The listing builds one solid part. Answer for the finished solid, in the listing's coordinates (mm). A direction names the side the tool comes from. Round coordinates to 2 decimals unless told otherwise and drop trailing zeros. Write each loop counter-clockwise with the first axis right and the second up, starting at its lowest first coordinate (ties: lowest second). Pieces come first, ordered by that corner, then holes. Notation, with made-up numbers: (28.5, 30) - (38.5, 30) arc R29 cw to (38.5, 67) - close; hole circle Ø5 at (52.5, 16.5). An arc over 180 degrees is marked (long way). Return JSON: item names as keys, results as strings. Group by question number.
(1) Each of these flat-tipped pins is pushed along its axis until it touches: pin 1 (3 mm diameter, centred on x = -20.5, z = 12.5, fed in from -Y); pin 2 (6 mm diameter, centred on x = -13, z = 32.5, fed in from -Y); pin 3 (1.7 mm diameter, centred on y = -5.5, z = 8, fed in from +X); pin 4 (5 mm diameter, centred on y = -9.5, z = 17, fed in from -X). Where does it stop, or does it pass through?
(2) Section A-A, the plane x = -32 is taken. Write down the section's boundary in (y, z), then the cut area to 3 significant figures.
(3) Section C-C, the plane x = -14.5 is taken. Write down the section's boundary in (y, z), then the cut area to 3 significant figures.
(4) Section D-D, the plane y = -5.5 is taken. Write down the section's boundary in (x, z).
(5) Find the intervals of material crossed by line 1 along Z through (x, y) = (-5.5, -13); line 2 along X through (y, z) = (-30, 10.5); line 3 along Z through (x, y) = (-29.5, -15), in increasing order. Write a range as [from, to].
(6) Which of the six approach directions +Z, -Z, +X, -X, +Y, -Y give full straight-line access (tool end or side, diameter ignored) to faces 4 (the flat face through (-5.317, -15, 28)), 5 (the flat face through (-15.106, -5.881, 5.82)), 6 (the flat face through (-15.028, -11, 14)), 7 (the flat face through (-4.28, -15.1, 23.88))?
(7) Determine the mould class of faces 1 (the flat face through (0, -28.7, 18.6)), 2 (the flat face through (-19.317, -6.287, 15.083)), 3 (the flat face through (-26.67, -6, 6)) for opening direction X: +X half, -X half, draft (parallel to the pull), parting line (faces both ways), or undercut.
(8) Section B-B, the plane z = 31 is taken. Write down the section's boundary in (x, y).
```python
from build123d import *

# Parameters (mm, degrees)
F0_W     = 38.1
F0_H     = 38.1
F1_DEPTH = 38.1
F4_W     = 21.59
F4_H     = 11.43
F5_DEPTH = 38.1
F7_DEPTH = 38.1
F8_W     = 20.69306
F8_H     = 6.94398
F9_DEPTH = 38.1


with BuildPart() as f1:
    # F0 (on Front) → F1 (new body)
    with BuildSketch(Plane.XZ):
        with Locations((-19.05, 19.05)):
            Rectangle(F0_W, F0_H)
    extrude(amount=F1_DEPTH)

    # F4 (on offset) → F5 (cut)
    with BuildSketch(Plane.XZ.offset(38.1)):
        with Locations((-16.112197, 27.854883)):
            Rectangle(F4_W, F4_H)
        Polygon((-26.67, 15.24), (-26.67, 0), (-16.748283, 0), (-12.880538, 0), (-7.961732, 0), align=None)
        Polygon((0, 4.241477), (0, 15.24), (-13.97, 15.24), align=None)
    extrude(amount=-F5_DEPTH, mode=Mode.SUBTRACT)

    # F6 (on offset) → F7 (cut)
    with BuildSketch(Plane.YZ.offset(-38.1)):
        Polygon((0, 38.1), (-12.885808, 38.1), (-1.962553, 0), (0, 0), align=None)
        Polygon((-18.980795, 31.710041), (-23.886719, 19.05), (-12.708837, 19.05), align=None)
        Polygon((-25.585808, 38.1), (-38.1, 38.1), (-38.1, 0), (-32.347631, 0), align=None)
        Polygon((-24.083182, 10.16), (-26.149293, 0), (-13.001305, 0), (-7.481929, 0), (-11.383182, 10.16), align=None)
    extrude(amount=F7_DEPTH, mode=Mode.SUBTRACT)

    # F8 (on Top) → F9 (cut)
    with BuildSketch(Plane.XY):
        Polygon((-15.027703, -7.71672), (-38.1, -7.71672), (-38.1, -12.706961), (-38.1, -14.533657), (-15.027703, -14.533657), align=None)
        with Locations((-10.34653, -24.610928)):
            Rectangle(F8_W, F8_H)
    extrude(amount=F9_DEPTH, mode=Mode.SUBTRACT)


solid = f1.part
```
Working result:
{
 "1": {"pin 1": "stops at y = -30.4", "pin 2": "stops at y = -21.14", "pin 3": "stops at x = -3.69", "pin 4": "stops at x = -38.1"},
 "2": {"outline": "(-32.35, 0) - (-26.15, 0) - (-24.08, 10.16) - (-14.53, 10.16) - (-14.53, 19.05) - (-23.89, 19.05) - (-18.98, 31.71) - (-14.53, 22.73) - (-14.53, 38.1) - (-25.59, 38.1) - close; (-7.72, 0.61) - (-7.48, 0) - (-1.96, 0) - (-7.72, 20.07) - close", "area": "433 mm^2"},
 "3": {"outline": "(-31.4, 5.33) - (-28.08, 5.33) - (-28.08, 22.14) - (-28.42, 22.14) - close; (-21.14, 10.16) - (-11.38, 10.16) - (-9.53, 5.33) - (-3.49, 5.33) - (-8.31, 22.14) - (-14.24, 22.14) - (-12.71, 19.05) - (-21.14, 19.05) - close; (-21.14, 33.57) - (-11.59, 33.57) - (-12.89, 38.1) - (-21.14, 38.1) - close", "area": "252 mm^2"},
 "4": {"outline": "(-38.1, 0) - (-26.67, 0) - (-26.67, 12.34) - (-38.1, 12.34) - close; (-23.11, 12.34) - (-7.96, 0) - (0, 0) - (0, 4.24) - (-10.28, 12.34) - close"},
 "5": {"line 1": "z = [15.24, 19.05], [19.64, 22.14], [33.57, 38.1]", "line 2": "x = [-38.1, -26.67], [-20.85, -7.95]", "line 3": "z = [10.16, 19.05], [23.67, 38.1]"},
 "6": {"face 4": "+Y, -Y", "face 5": "-Z, +Y, -Y", "face 6": "+Z, -Z, -X", "face 7": "+X, -X"},
 "7": {"face 1": "+X half", "face 2": "draft", "face 3": "undercut"},
 "8": {"outline": "(-38.1, -26.85) - (-26.91, -26.85) - (-26.91, -19.26) - (-38.1, -19.26) - close; (-38.1, -18.63) - (-26.91, -18.63) - (-26.91, -14.53) - (-38.1, -14.53) - close; (-5.32, -21.14) - (0, -21.14) - (0, -19.26) - (-5.32, -19.26) - close; (-5.32, -18.63) - (0, -18.63) - (0, -10.85) - (-5.32, -10.85) - close"}
}
